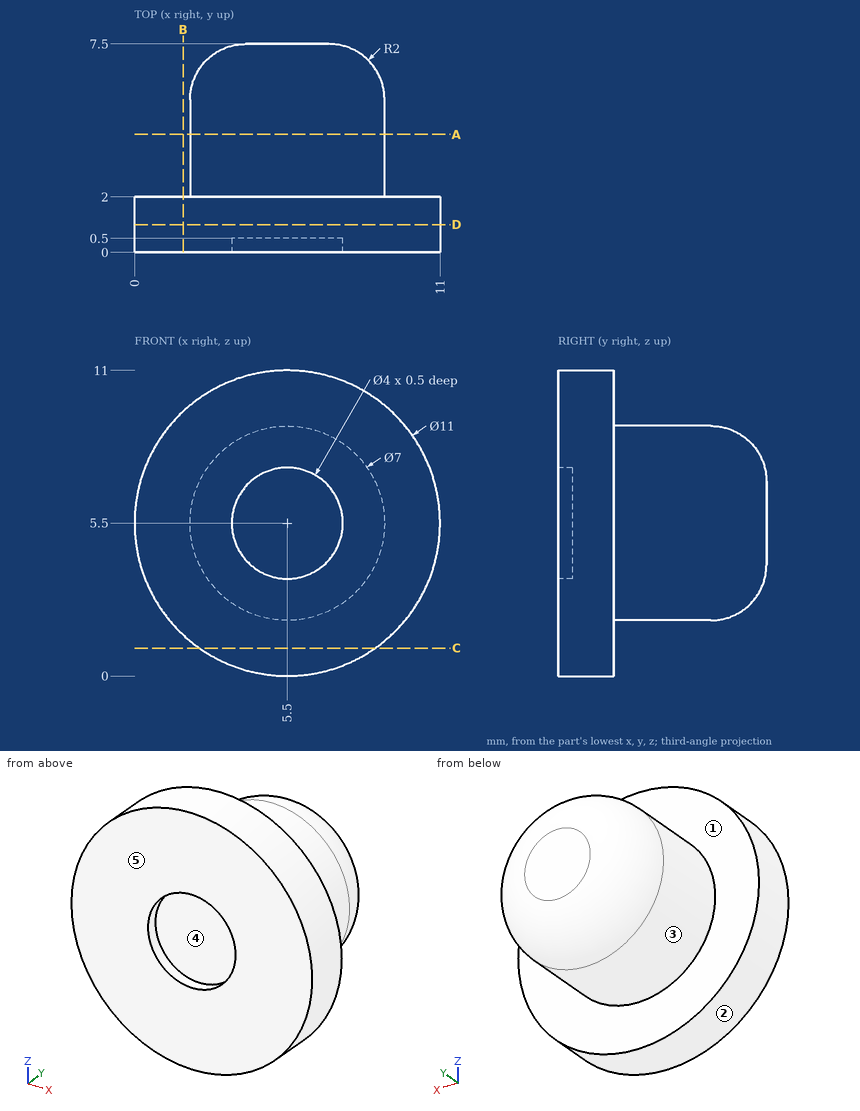
The figure shows three views and two pictorial views of one solid part (mm, origin at its lowest corner). Answer the questions. A direction names the side the tool comes from. Coordinates: 2 decimals unless noted, no trailing zeros. Order: outer loops, then holes, each group sorted by start corner. A loop starts at its lowest first (then second) coordinate and runs counter-clockwise, first axis right, second up.
Q1. Given P1, Ø1, axis at x = 2.5, y = 5, coming from the -Z side; P2, Ø2, axis at y = 2.5, z = 8, coming from the +X side, each flat-ended and moving along its own axis, determine where each tip first touches the part or whether it passes through.
Q2. A cutting plane is placed at A-A, the plane y = 4.25. Write down the section's boundary in (x, z).
Q3. For a pull along Z with two mould halves and no side action, classify the marked faces 3, 4 and 5 as pulls with the +Z half, pulls with the -Z half, needs draft (parallel to the pull), parting line crosses it, or undercut.
Q4. Which of the six approach directions +Z, -Z, +X, -X, +Y, -Y give full straight-line access (tool end or side, diameter ignored) to the marked faces 1 and 2?
Q5. A cutting plane is placed at C-C, the plane z = 1. Write down the section's boundary in (x, y), and give its area (3 significant figures).
Q6. A cutting plane is placed at B-B, the plane x = 1.75. Write down the section's boundary in (y, z), and give its area (3 significant figures).
Q7. A cutting plane is placed at D-D, the plane y = 1. Write down the section's boundary in (x, z), and give its area (3 significant figures).
Q8. Consider line 1 (Y direction, x = 10.25, z = 4); line 2 (Z direction, x = 5.5, y = 0.25); line 3 (Z direction, x = 5.5, y = 5.25). Determine where each line is inside the solid, lowest interval first.
Answers follow:
1. P1: stops at z = 3.05
1. P2: stops at x = 10.75
2. outline: circle Ø7 at (5.5, 5.5)
3. face 3: parting line crosses it
3. face 4: undercut
3. face 5: needs draft
4. face 1: +Y
4. face 2: +Y, -Y
5. outline: (2.34, 0) - (8.66, 0) - (8.66, 2) - (2.34, 2) - close
5. area: 12.6 mm2
6. outline: (0, 1.48) - (2, 1.48) - (2, 9.52) - (0, 9.52) - close
6. area: 16.1 mm2
7. outline: circle Ø11 at (5.5, 5.5)
7. area: 95.0 mm2
8. line 1: y = 0 to 2
8. line 2: z = 0 to 3.5, 7.5 to 11
8. line 3: z = 2 to 9
